Geometry check sheet. Reference: the model listing, model coordinates, mm. Round coordinates to 2 decimals unless told otherwise and drop trailing zeros. Loops run counter-clockwise (first coordinate to the right, second up) from the corner with the lowest first, then second, coordinate; pieces in that order, holes last. Notation, with made-up numbers: (0, -34) - (17, -34) arc R25 cw to (17, 1) - close; hole circle Ø2 at (19.5, 5). An arc over 180 degrees is marked (long way). Answer as CSV lines item,"result". Start each with the question number.
1) Cross-section at A-A on x = 12.7. Record the boundary of the cut face in (y, z) (3 decimals).
2) Depth check by flat-ended pin: P1, Ø4.5, axis at x = 75.74, y = -11, coming from the -Z side; P2, Ø1.6, axis at y = 67.5, z = 2, coming from the +X side; P3, Ø1.5, axis at y = 34, z = 2, coming from the +X side; P4, Ø1, axis at x = 19, z = 1, coming from the -Y side. Enter the tip coordinate at first touch or a pass-through.
3) Draft check along Y on faces 1 (the flat face through (52.69, -21.87, 1.57)), 2 (the flat face through (13, 76.2, 2)), 3 (the cylindrical face through (48.01, 9.45, 1.57)), 4 (the cylindrical face through (51.495, -3.558, 1.565)). Enter one of: released by +Y, released by -Y, zero draft, split by the parting line, or undercut.
4) Cross-section at B-B on y = 38.1. Record the boundary of the cut face in (x, z) (3 decimals).
5) Cross-section at C-C on x = 38. Record the boundary of the cut face in (y, z) (1 decimal), and give its area (3 significant figures).
6) Cross-section at D-D on z = 1.2. State how many separate pieces and enclosed holes the cut face has, and give its area (3 significant figures).
7) Thickness scan on line 1 along Y through (x, z) = (12.7, 2.15); line 2 along Y through (x, z) = (57, 1.85); line 3 along Y through (x, z) = (9, 1.3). Record the ranges inside material, lowest first.
from build123d import *

# Parameters (mm, degrees)
SKETCH1_R           = 2.5527
BOSS_EXTRUDE1_DEPTH = 3.175


with BuildPart() as part:
    # Sketch1 → Boss-Extrude1 (new body)
    with BuildSketch(Plane(origin=(0, 0, 0), x_dir=(-1, 0, 0), z_dir=(0, 0, -1))):
        with BuildLine():
            Line((-4.414213562, 0.585786438), (-0.585786438, 4.414213562))
            ThreePointArc((-0.585786438, 4.414213562), (-0.152240935, 5.06306026), (0, 5.828427125))
            Line((0, 5.828427125), (0, 70.371572875))
            ThreePointArc((0, 70.371572875), (-0.152240935, 71.13693974), (-0.585786438, 71.785786438))
            Line((-0.585786438, 71.785786438), (-4.414213562, 75.614213562))
            ThreePointArc((-4.414213562, 75.614213562), (-5.06306026, 76.047759065), (-5.828427125, 76.2))
            Line((-5.828427125, 76.2), (-19.571572875, 76.2))
            ThreePointArc((-19.571572875, 76.2), (-20.33693974, 76.047759065), (-20.985786438, 75.614213562))
            Line((-20.985786438, 75.614213562), (-24.814213562, 71.785786438))
            ThreePointArc((-24.814213562, 71.785786438), (-25.247759065, 71.13693974), (-25.4, 70.371572875))
            Line((-25.4, 70.371572875), (-25.4, 65.998533312))
            ThreePointArc((-25.4, 65.998533312), (-25.570370869, 64.704438086), (-26.069872981, 63.498533312))
            Line((-26.069872981, 63.498533312), (-29.926279442, 56.819041388))
            ThreePointArc((-29.926279442, 56.819041388), (-30.720872555, 55.783507482), (-31.756406461, 54.988914369))
            Line((-31.756406461, 54.988914369), (-91.840638796, 20.299266656))
            ThreePointArc((-91.840638796, 20.299266656), (-93.04654357, 19.799764543), (-94.340638796, 19.629393675))
            Line((-94.340638796, 19.629393675), (-102.053451717, 19.629393675))
            ThreePointArc((-102.053451717, 19.629393675), (-103.347546942, 19.799764543), (-104.553451717, 20.299266656))
            Line((-104.553451717, 20.299266656), (-108.34061507, 22.485786438))
            ThreePointArc((-108.34061507, 22.485786438), (-109.079562686, 22.736625353), (-109.858253161, 22.685587283))
            Line((-109.858253161, 22.685587283), (-115.08798187, 21.284285698))
            ThreePointArc((-115.08798187, 21.284285698), (-115.787866637, 20.939140726), (-116.302394587, 20.352434046))
            Line((-116.302394587, 20.352434046), (-123.173967462, 8.450520698))
            ThreePointArc((-123.173967462, 8.450520698), (-123.424806377, 7.711573082), (-123.373768307, 6.932882608))
            Line((-123.373768307, 6.932882608), (-121.972466723, 1.703153899))
            ThreePointArc((-121.972466723, 1.703153899), (-121.627321751, 1.003269131), (-121.04061507, 0.488741182))
            Line((-121.04061507, 0.488741182), (-65.14461121, -31.782831694))
            ThreePointArc((-65.14461121, -31.782831694), (-64.405663595, -32.033670609), (-63.62697312, -31.982632539))
            Line((-63.62697312, -31.982632539), (-58.397244411, -30.581330955))
            ThreePointArc((-58.397244411, -30.581330955), (-57.697359643, -30.236185983), (-57.182831694, -29.649479302))
            Line((-57.182831694, -29.649479302), (-48.066918237, -13.860254038))
            ThreePointArc((-48.066918237, -13.860254038), (-47.272325124, -12.824720132), (-46.236791218, -12.030127019))
            Line((-46.236791218, -12.030127019), (-26.560254038, -0.669872981))
            ThreePointArc((-26.560254038, -0.669872981), (-25.354349263, -0.170370869), (-24.060254038, 0))
            Line((-24.060254038, 0), (-5.828427125, 0))
            ThreePointArc((-5.828427125, 0), (-5.06306026, 0.152240935), (-4.414213562, 0.585786438))
        make_face()
        with Locations((-33.792281133, 16.076625677)):
            Circle(SKETCH1_R, mode=Mode.SUBTRACT)
        with Locations((-57.123670933, 2.606241495)):
            Circle(SKETCH1_R, mode=Mode.SUBTRACT)
        with Locations((-32.446584062, 5.855041615)):
            Circle(SKETCH1_R, mode=Mode.SUBTRACT)
        with Locations((-48.944368004, -3.669958385)):
            Circle(SKETCH1_R, mode=Mode.SUBTRACT)
        with Locations((-12.7, 12.7)):
            Circle(SKETCH1_R, mode=Mode.SUBTRACT)
        with Locations((-12.7, 38.1)):
            Circle(SKETCH1_R, mode=Mode.SUBTRACT)
        with Locations((-12.7, 63.5)):
            Circle(SKETCH1_R, mode=Mode.SUBTRACT)
        with Locations((-64.745567884, -17.348522628)):
            Circle(SKETCH1_R, mode=Mode.SUBTRACT)
        with Locations((-86.74261314, -4.648522628)):
            Circle(SKETCH1_R, mode=Mode.SUBTRACT)
        with Locations((-108.739658396, 8.051477372)):
            Circle(SKETCH1_R, mode=Mode.SUBTRACT)
        with Locations((-12.7, 25.4)):
            Circle(SKETCH1_R, mode=Mode.SUBTRACT)
        with Locations((-12.7, 50.8)):
            Circle(SKETCH1_R, mode=Mode.SUBTRACT)
        with Locations((-75.744090512, -10.998522628)):
            Circle(SKETCH1_R, mode=Mode.SUBTRACT)
        with Locations((-97.741135768, 1.701477372)):
            Circle(SKETCH1_R, mode=Mode.SUBTRACT)
        with Locations((-41.971584062, 22.352825557)):
            Circle(SKETCH1_R, mode=Mode.SUBTRACT)
        with Locations((-58.469368004, 12.827825557)):
            Circle(SKETCH1_R, mode=Mode.SUBTRACT)
        with Locations((-45.457976033, 9.341433586)):
            Circle(SKETCH1_R, mode=Mode.SUBTRACT)
        with Locations((-38.722783942, -2.324261314)):
            Circle(SKETCH1_R, mode=Mode.SUBTRACT)
        with BuildLine():
            Line((-54.403871172, 19.730778486), (-57.193679081, 24.562867528))
            ThreePointArc((-57.193679081, 24.562867528), (-56.259326033, 28.049920576), (-52.772272985, 27.115567528))
            Line((-52.772272985, 27.115567528), (-49.982465075, 22.283478486))
            ThreePointArc((-49.982465075, 22.283478486), (-50.916818124, 18.796425438), (-54.403871172, 19.730778486))
        make_face(mode=Mode.SUBTRACT)
    extrude(amount=-BOSS_EXTRUDE1_DEPTH)


solid = part.part
Answer block:
1,outline,"(0, 0) - (10.147, 0) - (10.147, 3.175) - (0, 3.175) - close; (15.253, 0) - (22.847, 0) - (22.847, 3.175) - (15.253, 3.175) - close; (27.953, 0) - (35.547, 0) - (35.547, 3.175) - (27.953, 3.175) - close; (40.653, 0) - (48.247, 0) - (48.247, 3.175) - (40.653, 3.175) - close; (53.353, 0) - (60.947, 0) - (60.947, 3.175) - (53.353, 3.175) - close; (66.053, 0) - (76.2, 0) - (76.2, 3.175) - (66.053, 3.175) - close"
2,P1,"passes through"
2,P2,"stops at x = 25.4"
2,P3,"stops at x = 69.41"
2,P4,"stops at y = 0"
3,face 1,"released by -Y"
3,face 2,"released by +Y"
3,face 3,"undercut"
3,face 4,"undercut"
4,outline,"(0, 0) - (10.147, 0) - (10.147, 3.175) - (0, 3.175) - close; (15.253, 0) - (61.009, 0) - (61.009, 3.175) - (15.253, 3.175) - close"
5,outline,"(-7.3, 0) - (-4.8, 0) - (-4.8, 3.2) - (-7.3, 3.2) - close; (0.1, 0) - (51.4, 0) - (51.4, 3.2) - (0.1, 3.2) - close"
5,area,"171 mm^2"
6,separate pieces,"1"
6,enclosed holes,"19"
6,area,"6,190 mm^2"
7,line 1,"y = 0 to 10.15, 15.25 to 22.85, 27.95 to 35.55, 40.65 to 48.25, 53.35 to 60.95, 66.05 to 76.2"
7,line 2,"y = -29.33 to 0.06, 5.16 to 10.74, 14.92 to 24.23, 27.4 to 40.41"
7,line 3,"y = 0 to 76.2"
